```python
from build123d import *

# Parameters (mm, degrees)
EXTRUDE1_DEPTH = 28.75
EXTRUDE2_START = 18.75
SKETCH2_R      = 2
EXTRUDE2_DEPTH = 3
EXTRUDE3_START = -15.75
SKETCH_R       = 2
EXTRUDE3_DEPTH = 3


with BuildPart() as part:
    # Sketch1 → Extrude1 (new, symmetric)
    with BuildSketch(Plane(origin=(0, 0, 0), x_dir=(0, 0, -1), z_dir=(1, 0, 0))):
        with BuildLine():
            Line((-6, 0), (-20, 0))
            Line((-20, 0), (-20, -20))
            Line((-20, -20), (0, -20))
            Line((0, -20), (0, -6))
            ThreePointArc((0, -6), (-1.757359313, -1.757359313), (-6, 0))
        make_face()
    extrude(amount=EXTRUDE1_DEPTH, both=True)

    # Sketch2 → Extrude2 (add)
    with BuildSketch(Plane(origin=(0, 0, 0), x_dir=(0, 0, -1), z_dir=(1, 0, 0)).offset(EXTRUDE2_START)):
        with BuildLine():
            Line((-6.707106781, -14.485281374), (10.970562748, 3.192388155))
            ThreePointArc((10.970562748, 3.192388155), (10.970562748, 10.970562748), (3.192388155, 10.970562748))
            Line((3.192388155, 10.970562748), (-14.485281374, -6.707106781))
            Line((-14.485281374, -6.707106781), (-6.707106781, -14.485281374))
        make_face()
        with Locations((7.081475452, 7.081475452)):
            Circle(SKETCH2_R, mode=Mode.SUBTRACT)
    extrude(amount=-EXTRUDE2_DEPTH)

    # Sketch → Extrude3 (add)
    with BuildSketch(Plane(origin=(0, 0, 0), x_dir=(0, 0, -1), z_dir=(1, 0, 0)).offset(EXTRUDE3_START)):
        with BuildLine():
            Line((-6.707106781, -14.485281374), (10.970562748, 3.192388155))
            ThreePointArc((10.970562748, 3.192388155), (10.970562748, 10.970562748), (3.192388155, 10.970562748))
            Line((3.192388155, 10.970562748), (-14.485281374, -6.707106781))
            Line((-14.485281374, -6.707106781), (-6.707106781, -14.485281374))
        make_face()
        with Locations((7.081475452, 7.081475452)):
            Circle(SKETCH_R, mode=Mode.SUBTRACT)
    extrude(amount=-EXTRUDE3_DEPTH)


solid = part.part
```
The listing builds one solid part. Answer for the finished solid, in the listing's coordinates (mm). A direction names the side the tool comes from. Give positions to 0.01 mm unless a question says otherwise; leave off trailing zeros. Loops run counter-clockwise (first coordinate to the right, second up) from the corner with the lowest first, then second, coordinate; pieces in that order, holes last. Notation, with made-up numbers: (12, -30.5) - (25, -30.5) arc R21 cw to (25, 1.5) - close; hole circle Ø11 at (61, 63). An arc over 180 degrees is marked (long way). Return JSON: item names as keys, results as strings. Group by question number.
1. Determine the mould class of faces 1 (the flat face through (-15.75, 5, -2)), 2 (the flat face through (-17.23, 5.56, 2.22)), 3 (the cylindrical face through (-17.229, 5.307, -8.004)) for opening direction Y: pulls with the +Y half, pulls with the -Y half, needs draft (parallel to the pull), parting line crosses it, or undercut.
2. Find section D-D (x = 0.5). Write down the section's boundary in (y, z), then the cut area to 3 significant figures.
3. Which of the six approach directions +Z, -Z, +X, -X, +Y, -Y give full straight-line access (tool end or side, diameter ignored) to faces 4 (the flat face through (0, -20, 10)), 5 (the cylindrical face through (-17.23, 10.88, -11.06)), 6 (the cylindrical face through (-23.68, -1.804, 1.711)), 7 (the flat face through (18.75, 5, -2)), 8 (the cylindrical face through (0.22, -1.804, 1.711))?
4. Find section A-A (y = 1). Write down the section's boundary in (x, z).
5. Find section C-C (z = 16.5). Write down the section's boundary in (x, y), then the cut area to 3 significant figures.
6. Straight lines are drawn through the part: line 1 (X direction, y = 10.5, z = -7); line 2 (Z direction, x = 22, y = -14); line 3 (Y direction, x = -21.5, z = 18). For each, find the intervals that lie inside material, in ascending order. Write a range as [from, to].
7. Given pin 1 Ø7 at (x, y) = (10, -9.5) entering from -Z; pin 2 Ø6 at (x, z) = (21, 8) entering from +Y; pin 3 Ø12 at (x, z) = (17, 11.5) entering from +Y, each flat-ended and moving along its own axis, determine where each tip first touches the part or whether it passes through.
8. Find section B-B (y = 6). Write down the section's boundary in (x, z).
Verdict:
{
 "1": {"face 1": "needs draft", "face 2": "pulls with the +Y half", "face 3": "undercut"},
 "2": {"outline": "(-20, 0) - (-6, 0) arc R6 ccw to (0, 6) - (0, 20) - (-20, 20) - close", "area": "392 mm^2"},
 "3": {"face 4": "+Z, -Z, +X, -X, -Y", "face 5": "+X, -X", "face 6": "-Z, -X, +Y", "face 7": "-Z, +X, +Y", "face 8": "-Z, +Y"},
 "4": {"outline": "(-18.75, -8.78) - (-15.75, -8.78) - (-15.75, 6.78) - (-18.75, 6.78) - close; (15.75, -8.78) - (18.75, -8.78) - (18.75, 6.78) - (15.75, 6.78) - close"},
 "5": {"outline": "(-28.75, -20) - (28.75, -20) - (28.75, 0) - (-28.75, 0) - close", "area": "1,150 mm^2"},
 "6": {"line 1": "x = [-18.75, -15.75], [15.75, 18.75]", "line 2": "z = [0, 20]", "line 3": "y = [-20, 0]"},
 "7": {"pin 1": "stops at z = 0", "pin 2": "stops at y = 1.76", "pin 3": "stops at y = 2.28"},
 "8": {"outline": "(-18.75, -12.47) - (-15.75, -12.47) - (-15.75, -8.76) - (-18.75, -8.76) - close; (-18.75, -5.4) - (-15.75, -5.4) - (-15.75, 1.78) - (-18.75, 1.78) - close; (15.75, -12.47) - (18.75, -12.47) - (18.75, -8.76) - (15.75, -8.76) - close; (15.75, -5.4) - (18.75, -5.4) - (18.75, 1.78) - (15.75, 1.78) - close"}
}
